```python
from build123d import *

# Parameters (mm, degrees)
AUFSATZ_LINEAR_AUSTRAGEN1_DEPTH = 480
SKIZZE2_R                       = 2.75
SCHNITT_LINEAR_AUSTRAGEN1_DEPTH = 100
SKIZZE3_R                       = 2.75
SCHNITT_LINEAR_AUSTRAGEN2_DEPTH = 100
SKIZZE4_R                       = 2.5
SCHNITT_LINEAR_AUSTRAGEN3_DEPTH = 100
SKIZZE5_R                       = 2.5
SCHNITT_LINEAR_AUSTRAGEN4_DEPTH = 100


with BuildPart() as part:
    # Skizze1 → Aufsatz-Linear austragen1 (new, symmetric)
    with BuildSketch(Plane.XY):
        with BuildLine():
            Line((-34, 20), (34, 20))
            ThreePointArc((34, 20), (38.242640687, 18.242640687), (40, 14))
            Line((40, 14), (40, -14))
            ThreePointArc((40, -14), (38.242640687, -18.242640687), (34, -20))
            Line((34, -20), (-34, -20))
            ThreePointArc((-34, -20), (-38.242640687, -18.242640687), (-40, -14))
            Line((-40, -14), (-40, 14))
            ThreePointArc((-40, 14), (-38.242640687, 18.242640687), (-34, 20))
        make_face()
        with BuildLine():
            Line((-38, 14), (-38, -14))
            ThreePointArc((-38, -14), (-36.828427125, -16.828427125), (-34, -18))
            Line((-34, -18), (34, -18))
            ThreePointArc((34, -18), (36.828427125, -16.828427125), (38, -14))
            Line((38, -14), (38, 14))
            ThreePointArc((38, 14), (36.828427125, 16.828427125), (34, 18))
            Line((34, 18), (-34, 18))
            ThreePointArc((-34, 18), (-36.828427125, 16.828427125), (-38, 14))
        make_face(mode=Mode.SUBTRACT)
    extrude(amount=AUFSATZ_LINEAR_AUSTRAGEN1_DEPTH, both=True)

    # Skizze2 → Schnitt-Linear austragen1 (cut)
    with BuildSketch(Plane(origin=(0, 20, 0), x_dir=(1, 0, 0), z_dir=(0, 1, 0))):
        with Locations(Location((20, 460, 0), (0, 0, 270))):
            Circle(SKIZZE2_R)
        with Locations((-20, 460)):
            Circle(SKIZZE2_R)
        with Locations((20, -460)):
            Circle(SKIZZE2_R)
        with Locations(Location((-20, -460, 0), (0, 0, 270))):
            Circle(SKIZZE2_R)
    extrude(amount=-SCHNITT_LINEAR_AUSTRAGEN1_DEPTH, mode=Mode.SUBTRACT)

    # Skizze3 → Schnitt-Linear austragen2 (cut)
    with BuildSketch(Plane(origin=(40, 0, 0), x_dir=(0, 0, -1), z_dir=(1, 0, 0))):
        with Locations((460, 0)):
            Circle(SKIZZE3_R)
        with Locations(Location((-460, 0, 0), (0, 0, 270))):
            Circle(SKIZZE3_R)
    extrude(amount=-SCHNITT_LINEAR_AUSTRAGEN2_DEPTH, mode=Mode.SUBTRACT)

    # Skizze4 → Schnitt-Linear austragen3 (cut)
    with BuildSketch(Plane(origin=(40, 0, 0), x_dir=(0, 0, -1), z_dir=(1, 0, 0))):
        with Locations((-270, 0)):
            Circle(SKIZZE4_R)
        with Locations((-90, 0)):
            Circle(SKIZZE4_R)
        with Locations(Location((90, 0, 0), (0, 0, 270))):
            Circle(SKIZZE4_R)
        with Locations(Location((270, 0, 0), (0, 0, 270))):
            Circle(SKIZZE4_R)
    extrude(amount=-SCHNITT_LINEAR_AUSTRAGEN3_DEPTH, mode=Mode.SUBTRACT)

    # Skizze5 → Schnitt-Linear austragen4 (cut)
    with BuildSketch(Plane(origin=(0, 20, 0), x_dir=(1, 0, 0), z_dir=(0, 1, 0))):
        with Locations(Location((20, 270, 0), (0, 0, 270))):
            Circle(SKIZZE5_R)
        with Locations(Location((20, 90, 0), (0, 0, 270))):
            Circle(SKIZZE5_R)
        with Locations((-20, 90)):
            Circle(SKIZZE5_R)
        with Locations((-20, 270)):
            Circle(SKIZZE5_R)
        with Locations((20, -90)):
            Circle(SKIZZE5_R)
        with Locations(Location((-20, -90, 0), (0, 0, 270))):
            Circle(SKIZZE5_R)
        with Locations((20, -270)):
            Circle(SKIZZE5_R)
        with Locations(Location((-20, -270, 0), (0, 0, 270))):
            Circle(SKIZZE5_R)
    extrude(amount=-SCHNITT_LINEAR_AUSTRAGEN4_DEPTH, mode=Mode.SUBTRACT)


solid = part.part
```
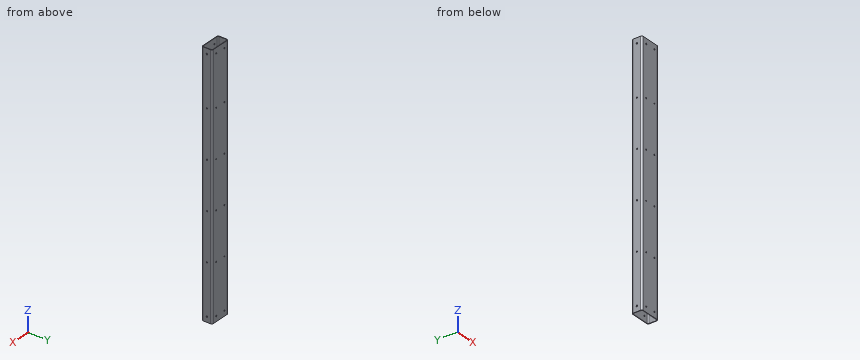
The listing builds one solid part. Answer for the finished solid, in the listing's coordinates (mm). Give positions to 0.01 mm unless a question says otherwise; leave off trailing zeros. Order: outer loops, then holes, each group sorted by start corner. A loop starts at its lowest first (then second) coordinate and runs counter-clockwise, first axis right, second up. Notation, with made-up numbers: (24.25, 18.25) -> (32.25, 18.25) arc R20 cw to (32.25, 22.25) -> close; hole circle Ø7 at (8.25, 86.5). An arc over 180 degrees is marked (long way). Write each question's results on one line, items separated by ' | '.
Q1. The part is cut by section B-B, the plane z = 250. Give the vertices of the cut face in (x, y).
Checked values:
outline: (-40, -14) arc R6 ccw to (-34, -20) -> (34, -20) arc R6 ccw to (40, -14) -> (40, 14) arc R6 ccw to (34, 20) -> (-34, 20) arc R6 ccw to (-40, 14) -> close; hole (-38, -14) arc R4 ccw to (-34, -18) -> (34, -18) arc R4 ccw to (38, -14) -> (38, 14) arc R4 ccw to (34, 18) -> (-34, 18) arc R4 ccw to (-38, 14) -> close
Q2. Straight lines are drawn through the part: probe 1 along X at (y, z) = (4, -259); probe 2 along Y at (x, z) = (-31.5, -190); probe 3 along X at (y, z) = (19, -90). For each, find the intervals that lie inside material, in ascending order. Write a range as from..to.
Checked values:
probe 1: x = -40..-38, 38..40 | probe 2: y = -20..-18, 18..20 | probe 3: x = -37.32..-22.5, -17.5..17.5, 22.5..37.32
Q3. This flat-tipped pin is pushed along its axis until it touches: P1, Ø3, axis at y = 0, z = 270, coming from the -X side. Where does it stop, or does it pass through?
Checked values:
P1: passes through
Q4. The part is cut by section A-A, the plane x = 8. Give the vertices of the cut face in (y, z), and give its area (3 significant figures).
Checked values:
outline: (-20, -480) -> (-18, -480) -> (-18, 480) -> (-20, 480) -> close; (18, -480) -> (20, -480) -> (20, 480) -> (18, 480) -> close | area: 3,840 mm^2
